```python
from build123d import *

# Parameters (mm, degrees)
BOSS_EXTRUDE1_DEPTH = 2
EDGE_FLANGE1_DEPTH  = 2
EDGE_FLANGE2_DEPTH  = 2
SKETCH13_W          = 2.5
SKETCH13_H          = 2.15
SKETCH13_W_2        = 3
CUT_EXTRUDE3_DEPTH  = 10


# Sheet-metal steps are written as plain solids
with BuildPart() as part:
    # Sketch2 → Boss-Extrude1 (new body)
    with BuildSketch(Plane(origin=(0, 0, 0), x_dir=(1, 0, 0), z_dir=(0, 1, 0))):
        Polygon((-52.543309772, 32.413356753), (-54.793309772, 32.413356753), (-54.793309772, 30.413356753), (64.413548219, 30.413356753), (67.959993108, 26.866911863), (67.959993108, 23.966910068), (75.359993548, 16.566912168), (75.359993548, -11.849150158), (67.759993508, -19.449150198), (67.759993508, -31.745752353), (62.750836838, -36.754909023), (58.359994528, -36.754909023), (58.359994528, -42.739906444), (71.753176861, -42.739906444), (75.659994488, -38.833088817), (75.659994488, -22.433088597), (81.359993248, -16.733089837), (81.359993248, 1.669814581), (83.609993248, 1.669814581), (83.609993248, 3.669814581), (81.359993248, 3.669814581), (81.359993248, 19.459804242), (66.106440177, 34.713357313), (-52.543309772, 34.713357313), align=None)
    extrude(amount=BOSS_EXTRUDE1_DEPTH)

    # Edge-Flange1 section (across the edge) → Edge-Flange1 (add)
    with BuildSketch(Plane(origin=(-55.793309772, 0, -30.413356753), x_dir=(1, 0, 0), z_dir=(0, 0, -1))):
        with BuildLine():
            Line((-2, 0.5), (-2, 1.4))
            Line((-2, 1.4), (0, 1.4))
            Line((0, 1.4), (0, 0.5))
            ThreePointArc((0, 0.5), (0.146446609, 0.146446609), (0.5, 0))
            Line((0.5, 0), (1, 0))
            Line((1, 0), (1, -2))
            Line((1, -2), (0.5, -2))
            ThreePointArc((0.5, -2), (-1.267766953, -1.267766953), (-2, 0.5))
        make_face()
    extrude(amount=EDGE_FLANGE1_DEPTH)

    # Edge-Flange2 section (across the edge) → Edge-Flange2 (add)
    with BuildSketch(Plane(origin=(84.609993248, 0, -3.669814581), x_dir=(-1, 0, 0), z_dir=(0, 0, 1))):
        with BuildLine():
            Line((-2, 0.5), (-2, 1.4))
            Line((-2, 1.4), (0, 1.4))
            Line((0, 1.4), (0, 0.5))
            ThreePointArc((0, 0.5), (0.146446609, 0.146446609), (0.5, 0))
            Line((0.5, 0), (1, 0))
            Line((1, 0), (1, -2))
            Line((1, -2), (0.5, -2))
            ThreePointArc((0.5, -2), (-1.267766953, -1.267766953), (-2, 0.5))
        make_face()
    extrude(amount=EDGE_FLANGE2_DEPTH)

    # Sketch13 → Cut-Extrude3 (cut)
    with BuildSketch(Plane(origin=(0, 2, 0), x_dir=(1, 0, 0), z_dir=(0, 1, 0))):
        with Locations((-27.730006168, 34.839358373)):
            Rectangle(SKETCH13_W, SKETCH13_H)
        with Locations((-42.672006168, 34.839358373)):
            Rectangle(SKETCH13_W_2, SKETCH13_H)
        with Locations((-12.490006168, 34.839358373)):
            Rectangle(SKETCH13_W, SKETCH13_H)
        with Locations((2.749993832, 34.839358373)):
            Rectangle(SKETCH13_W, SKETCH13_H)
        with Locations((17.608993832, 34.839358373)):
            Rectangle(SKETCH13_W, SKETCH13_H)
        with Locations((32.213993832, 34.839358373)):
            Rectangle(SKETCH13_W, SKETCH13_H)
        with Locations((47.453993832, 34.839358373)):
            Rectangle(SKETCH13_W, SKETCH13_H)
        with Locations((61.931993832, 34.839358373)):
            Rectangle(SKETCH13_W, SKETCH13_H)
    extrude(amount=-CUT_EXTRUDE3_DEPTH, mode=Mode.SUBTRACT)


solid = part.part
```
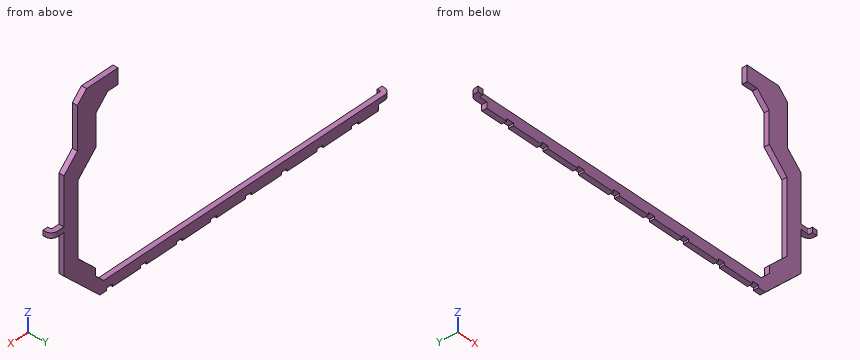
CAD build for the part. Positions are in the model's coordinates, mm. Round coordinates to 2 decimals unless told otherwise and drop trailing zeros. Order: outer loops, then holes, each group sorted by start corner. A loop starts at its lowest first (then second) coordinate and runs counter-clockwise, first axis right, second up.
Item 1: Pin check, flat tips, straight feed: pin 1 (2 mm diameter, centred on y = 1, z = -34, fed in from -X); pin 2 (1 mm diameter, centred on y = 1.5, z = -34, fed in from +X); pin 3 (0.6 mm diameter, centred on y = 1, z = 7.5, fed in from +X); pin 4 (23 mm diameter, centred on x = 30.5, z = -10.5, fed in from -Y). Stop position of each tip, or through.
Item 2: Saw through at B-B on x = 13. Write the cut outline in (y, z), then the cut area to 3 significant figures.
Item 3: Probe line 1 along Z through (x, y) = (13, 1.4); line 2 along X through (y, z) = (0.15, 29.5); line 3 along Y through (x, z) = (75, 35). List the from-to ranges inside material, lowest first.
Item 4: Saw through at A-A on z = -14. Write the cut outline in (x, y).
Reported:
1. pin 1: stops at x = -52.54
1. pin 2: stops at x = 67.32
1. pin 3: stops at x = 81.36
1. pin 4: passes through
2. outline: (0, -34.71) - (2, -34.71) - (2, -30.41) - (0, -30.41) - close
2. area: 8.60 mm2
3. line 1: z = -34.71 to -30.41
3. line 2: x = 67.76 to 75.66
3. line 3: y = 0 to 2
4. outline: (75.36, 0) - (81.36, 0) - (81.36, 2) - (75.36, 2) - close
